Geometry check sheet. Reference: the model listing, model coordinates, mm. Give positions to 0.01 mm unless a question says otherwise; leave off trailing zeros. Write each loop counter-clockwise with the first axis right and the second up, starting at its lowest first coordinate (ties: lowest second). Pieces come first, ordered by that corner, then holes.
(1) Thickness scan on line 1 along Y through (x, z) = (37, 0.45); line 2 along Y through (x, z) = (-9.5, 0.7); line 3 along Y through (x, z) = (73, 1.1). Record the ranges inside material, lowest first.
(2) Cross-section at A-A (y = -90). Record the boundary of the cut face in (x, z).
(3) Cross-section at B-B (x = -82.5). Record the boundary of the cut face in (y, z), and give its area (3 significant figures).
(4) Mould release check, pull along X, two halves, no side actions. Record for faces 1 (the cylindrical face through (-124.88, 5.5, 0.79)), 2 (the cylindrical face through (62.154, 2.253, 0.811)), 3 (the flat face through (-2, -26, 1.6)), 4 (the cylindrical face through (-2.38, -10.74, 0.81)): +X half, -X half, draft (parallel to the pull), parting line (faces both ways), or undercut.
```python
from build123d import *

# Parameters (mm, degrees)
SKETCH_1_R          = 125
EXTRUDE_1_DEPTH     = 1.6
SKETCH_2_R          = 11
CUT_EXTRUDE_1_DEPTH = 177.783935922
SKETCH_3_R          = 7.5
CUT_EXTRUDE_2_DEPTH = 177.783935922
M6X1_0_1_D          = 5
M6X1_0_2_D          = 5
M6X1_0_3_D          = 5
M6X1_0_4_D          = 5
M6X1_0_5_D          = 5
M6X1_0_6_D          = 5


with BuildPart() as part:
    # ｽｹｯﾁ1 → ﾎﾞｽ - 押し出し1 (new body)
    with BuildSketch(Plane.XY):
        Circle(SKETCH_1_R)
    extrude(amount=EXTRUDE_1_DEPTH)

    # ｽｹｯﾁ2 → ｶｯﾄ - 押し出し1 (cut, through all)
    with BuildSketch(Plane.XY.offset(1.6)):
        Circle(SKETCH_2_R)
    extrude(amount=-CUT_EXTRUDE_1_DEPTH, mode=Mode.SUBTRACT)

    # ｽｹｯﾁ3 → ｶｯﾄ - 押し出し2 (cut, through all)
    with BuildSketch(Plane.XY.offset(1.6)):
        with Locations((55, 0)):
            Circle(SKETCH_3_R)
    extrude(amount=-CUT_EXTRUDE_2_DEPTH, mode=Mode.SUBTRACT)

    # M6x1.0 ねじ穴1 (through all)
    with Locations(Plane(origin=(110, 0, 1.6), x_dir=(1, 0, 0), z_dir=(0, 0, 1))):
        with Locations((0, 0)):
            Hole(M6X1_0_1_D / 2)

    # M6x1.0 ねじ穴2 (through all)
    with Locations(Plane(origin=(-110, 0, 1.6), x_dir=(1, 0, 0), z_dir=(0, 0, 1))):
        with Locations((0, 0)):
            Hole(M6X1_0_2_D / 2)

    # M6x1.0 ねじ穴3 (through all)
    with Locations(Plane(origin=(-21, 0, 1.6), x_dir=(1, 0, 0), z_dir=(0, 0, 1))):
        with Locations((0, 0)):
            Hole(M6X1_0_3_D / 2)

    # M6x1.0 ねじ穴4 (through all)
    with Locations(Plane(origin=(21, 0, 1.6), x_dir=(1, 0, 0), z_dir=(0, 0, 1))):
        with Locations((0, 0)):
            Hole(M6X1_0_4_D / 2)

    # M6x1.0 ねじ穴5 (through all)
    with Locations(Plane(origin=(37, 18, 1.6), x_dir=(1, 0, 0), z_dir=(0, 0, 1))):
        with Locations((0, 0), (36, 0), (36, -36), (0, -36)):
            Hole(M6X1_0_5_D / 2)

    # M6x1.0 ねじ穴6 (through all)
    with Locations(Plane(origin=(0, 110, 1.6), x_dir=(1, 0, 0), z_dir=(0, 0, 1))):
        with Locations((0, 0), (0, -220)):
            Hole(M6X1_0_6_D / 2)


solid = part.part
```
Reply:
1. line 1: y = -119.4 to -20.5, -15.5 to 15.5, 20.5 to 119.4
1. line 2: y = -124.64 to -5.55, 5.55 to 124.64
1. line 3: y = -101.47 to -20.5, -15.5 to 15.5, 20.5 to 101.47
2. outline: (-86.75, 0) - (86.75, 0) - (86.75, 1.6) - (-86.75, 1.6) - close
3. outline: (-93.91, 0) - (93.91, 0) - (93.91, 1.6) - (-93.91, 1.6) - close
3. area: 301 mm2
4. face 1: parting line
4. face 2: undercut
4. face 3: draft
4. face 4: undercut
